Read the model definition and answer for the solid it produces. Units are mm, in the model's axes. Face numbers are marked on the shaded views. A direction names the side the tool comes from. Give positions to 0.01 mm unless a question says otherwise; leave off trailing zeros. Order: outer loops, then holes, each group sorted by start corner. A loop starts at its lowest first (then second) coordinate and runs counter-clockwise, first axis right, second up. Notation, with made-up numbers: (77, 36) - (122, 36) arc R9 cw to (122, 52) - close; hole circle Ø11 at (-28.75, -6.75). An arc over 180 degrees is marked (long way). Use a Markdown table: item, result. Add a question column.
1. A cutting plane is placed at A-A on z = 6.5. Determine the outline of the cut face in (x, y).
2. A cutting plane is placed at B-B on x = -31.5. Determine the outline of the cut face in (y, z), and give its area (3 significant figures).
3. For a pull along X with two mould halves and no side action, classify the marked faces 1, 2 and 3 as released by +X, released by -X, zero draft, split by the parting line, or undercut.
4. A cutting plane is placed at D-D on z = -19.5. Determine the outline of the cut face in (x, y), and give its area (3 significant figures).
5. Consider L1, parallel to X at y = 15, z = 1.5; L2, parallel to Y at x = -53.5, z = -22; L3, parallel to X at y = -77, z = 9.5. Determine where each line is inside the solid, lowest interval first.
6. Flat-ended cylindrical pins translate along their axes: P1, Ø3, axis at y = -39.5, z = 0.5, coming from the -X side; P2, Ø8, axis at x = 3, z = 5, coming from the -Y side; P3, Ø11, axis at y = -70, z = -20.5, coming from the -X side. Find the tip coordinate at first contact, or state that the pin passes through.
7. Which of the six approach directions +Z, -Z, +X, -X, +Y, -Y give full straight-line access (tool end or side, diameter ignored) to the marked faces 4, 5 and 6?
8. A cutting plane is placed at C-C on y = -66.5. Determine the outline of the cut face in (x, z), and give its area (3 significant figures).
```python
from build123d import *

# Parameters (mm, degrees)
F0_W          = 132.9678967595
F0_H          = 40.9901021048
F1_DEPTH      = 35.306
F2_W          = 109.3940883875
F2_H          = 52.1104875952
F3_DEPTH      = 57.15
F4_W          = 66.4839483798
F4_H          = 40.9901021048
F5_DEPTH      = 56.134
F6_W          = 53.8083352149
F6_H          = 26.0552437976
F7_DEPTH      = 59.69
F8_F1_R       = 5.08
F8_F2_R       = 5.08
F9_W          = 99.2340883875
F9_H          = 46.9125229284
F10_DEPTH     = 4.826
F11_W         = 43.6483352149
F11_H         = 56.2114770716
F12_DEPTH     = 4.826
F13_T1_DEPTH  = 56.3324502806
F13_T3_DEPTH  = 0.0774771487
F13_T5_DEPTH  = 68.8181149887
F13_T7_DEPTH  = 55.5857531726
F13_T9_DEPTH  = 115.8081150657
F13_T11_DEPTH = 99.2340883875
F13_T13_DEPTH = 59.5966379941
F13_T19_DEPTH = 68.2698682383
F13_T23_DEPTH = 12.7615922144


# Not quite as in the source:
# - a fillet or chamfer that OpenCascade refuses, or shapes differently, is made with other operations: its cross-section is extruded or revolved along the edge and cut away or added


with BuildPart() as f1:
    # F0 (on Front) → F1 (new body, symmetric)
    with BuildSketch(Plane.XZ):
        with Locations((0.8887089789, -5.8075287379)):
            Rectangle(F0_W, F0_H)
    extrude(amount=F1_DEPTH, both=True)

    # F2 (on face) → F3 (cut)
    with BuildSketch(Plane.XZ.offset(35.306)):
        with Locations((0, 14.6875223145)):
            Rectangle(F2_W, F2_H)
    extrude(amount=-F3_DEPTH, mode=Mode.SUBTRACT)

    # F4 (on face) → F5 (join)
    with BuildSketch(Plane.XZ.offset(35.306)):
        with Locations((34.1306831688, -5.8075287379)):
            Rectangle(F4_W, F4_H)
    extrude(amount=F5_DEPTH)

    # F6 (on face) → F7 (cut)
    with BuildSketch(Plane(origin=(0, -35.306, 0), x_dir=(-1, 0, 0), z_dir=(0, 1, 0))):
        with Locations((-27.7928765863, 1.6599004157)):
            Rectangle(F6_W, F6_H)
    extrude(amount=-F7_DEPTH, mode=Mode.SUBTRACT)

    # F8: fillet of radius 5.08 on 11 edges, made by hand

    # F8_f1
    f8_f1_edges = [f1.edges().sort_by_distance(p)[0] for p in [
        (-54.6970441937, -6.731, -11.3677214831),
        (-54.6970441937, 21.844, 1.6599004157),
        (0, 21.844, -11.3677214831),
        (54.6970441937, -34.798, -11.3677214831),
        (54.6970441937, 21.844, 1.6599004157),
    ]]
    fillet(f8_f1_edges, radius=F8_F1_R)

    # F8_f2
    f8_f2_edges = [f1.edges().sort_by_distance(p)[0] for p in [
        (-54.6970441937, -9.271, 14.6875223145),
        (0, 21.844, 14.6875223145),
        (54.6970441937, -37.338, 14.6875223145),
        (-24.3641676074, -35.306, -11.3677214831),
        (0.8887089789, -63.373, -11.3677214831),
        (25.2528765863, -91.44, -11.3677214831),
        (53.2091466422, -91.44, -9.8798239315),
        (-53.2091466422, -35.306, -9.8798239315),
        (53.2091466422, 20.3561024484, 14.6875223145),
        (-53.2091466422, 20.3561024484, 14.6875223145),
    ]]
    fillet(f8_f2_edges, radius=F8_F2_R)

    # F9 (on face) → F10 (join)
    with BuildSketch(Plane.XY.offset(-11.3677214831)):
        with Locations((0, -6.6922614642)):
            Rectangle(F9_W, F9_H)
    extrude(amount=F10_DEPTH)

    # F11 (on face) → F12 (join)
    with BuildSketch(Plane.XY.offset(-11.3677214831)):
        with Locations((27.7928765863, -58.2542614642)):
            Rectangle(F11_W, F11_H)
    extrude(amount=F12_DEPTH)

    # F13: fillet of radius 5.08 on 6 edges, made by hand

    # F13_s2 → F13_t1 (cut)
    with BuildSketch(Plane.YZ.offset(-6.7154060868)):
        with BuildLine():
            ThreePointArc((-81.2863539737, -6.5417214831), (-84.7875023567, -7.9409117896), (-86.36, -11.3677214831))
            Line((-86.36, -11.3677214831), (-86.36, -6.5417214831))
            Line((-86.36, -6.5417214831), (-81.2863539737, -6.5417214831))
        make_face()
    extrude(amount=F13_T1_DEPTH, mode=Mode.SUBTRACT)

    # F13_s4 → F13_t3 (cut)
    with BuildSketch(Plane.XZ.offset(30.1485229284)):
        with BuildLine():
            ThreePointArc((11.0423550052, -6.5417214831), (7.5412066221, -7.9409117896), (5.9687089789, -11.3677214831))
            Line((5.9687089789, -11.3677214831), (5.9687089789, -6.5417214831))
            Line((5.9687089789, -6.5417214831), (11.0423550052, -6.5417214831))
        make_face()
    extrude(amount=F13_T3_DEPTH, mode=Mode.SUBTRACT)

    # F13_s6 → F13_t5 (cut)
    with BuildSketch(Plane.XZ.offset(30.226000077)):
        with BuildLine():
            ThreePointArc((11.0423550052, -6.5417214831), (7.5412066221, -7.9409117896), (5.9687089789, -11.3677214831))
            Line((5.9687089789, -11.3677214831), (5.9687089789, -6.5417214831))
            Line((5.9687089789, -6.5417214831), (11.0423550052, -6.5417214831))
        make_face()
    extrude(amount=F13_T5_DEPTH, mode=Mode.SUBTRACT)

    # F13_s8 → F13_t7 (cut)
    with BuildSketch(Plane.YZ.offset(-49.6170441937)):
        with BuildLine():
            ThreePointArc((-25.0748769021, -6.5417214831), (-28.5760252851, -7.9409117896), (-30.1485229284, -11.3677214831))
            Line((-30.1485229284, -11.3677214831), (-30.1485229284, -6.5417214831))
            Line((-30.1485229284, -6.5417214831), (-25.0748769021, -6.5417214831))
        make_face()
    extrude(amount=F13_T7_DEPTH, mode=Mode.SUBTRACT)

    # F13_s10 → F13_t9 (cut)
    with BuildSketch(Plane.XZ.offset(-16.764)):
        with BuildLine():
            ThreePointArc((44.5433981675, -6.5417214831), (48.0445465505, -7.9409117896), (49.6170441937, -11.3677214831))
            Line((49.6170441937, -11.3677214831), (49.6170441937, -6.5417214831))
            Line((49.6170441937, -6.5417214831), (44.5433981675, -6.5417214831))
        make_face()
    extrude(amount=F13_T9_DEPTH, mode=Mode.SUBTRACT)

    # F13_s12 → F13_t11 (cut)
    with BuildSketch(Plane.YZ.offset(-49.6170441937)):
        with BuildLine():
            ThreePointArc((16.764, -11.3677214831), (15.1915023567, -7.9409117896), (11.6903539737, -6.5417214831))
            Line((11.6903539737, -6.5417214831), (16.764, -6.5417214831))
            Line((16.764, -6.5417214831), (16.764, -11.3677214831))
        make_face()
    extrude(amount=F13_T11_DEPTH, mode=Mode.SUBTRACT)

    # F13_s14 → F13_t13 (cut)
    with BuildSketch(Plane.XZ.offset(-16.764)):
        with BuildLine():
            ThreePointArc((-44.5433981675, -6.5417214831), (-48.0445465505, -7.9409117896), (-49.6170441937, -11.3677214831))
            Line((-49.6170441937, -11.3677214831), (-49.6170441937, -6.5417214831))
            Line((-49.6170441937, -6.5417214831), (-44.5433981675, -6.5417214831))
        make_face()
    extrude(amount=F13_T13_DEPTH, mode=Mode.SUBTRACT)


with BuildPart() as f13_tool17:
    # F13_s18 → F13_t19 (new body)
    with BuildSketch(Plane.YZ.offset(-49.6170441937)):
        with BuildLine():
            ThreePointArc((-25.0748769021, -6.5417214831), (-28.5760252851, -7.9409117896), (-30.1485229284, -11.3677214831))
            Line((-30.1485229284, -11.3677214831), (-30.1485229284, -6.5417214831))
            Line((-30.1485229284, -6.5417214831), (-25.0748769021, -6.5417214831))
        make_face()
    extrude(amount=F13_T19_DEPTH)

    split(bisect_by=Plane.YZ.offset(5.9687089789), keep=Keep.TOP)


with BuildPart() as f13_tool21:
    # F13_s22 → F13_t23 (new body)
    with BuildSketch(Plane.XZ.offset(17.4644078627)):
        with BuildLine():
            ThreePointArc((11.0423550052, -6.5417214831), (7.5412066221, -7.9409117896), (5.9687089789, -11.3677214831))
            Line((5.9687089789, -11.3677214831), (5.9687089789, -6.5417214831))
            Line((5.9687089789, -6.5417214831), (11.0423550052, -6.5417214831))
        make_face()
    extrude(amount=F13_T23_DEPTH)

    split(bisect_by=Plane.XZ.offset(30.1485229284), keep=Keep.BOTTOM)


with BuildPart() as f13_tool17_1:
    add(f13_tool17.part)

    # F13_t25: intersect F13_tool21
    add(f13_tool21.part, mode=Mode.INTERSECT)


with BuildPart() as f1_1:
    add(f1.part)

    # F13_t15: cut F13_tool17
    add(f13_tool17_1.part, mode=Mode.SUBTRACT)


solid = f1_1.part
```
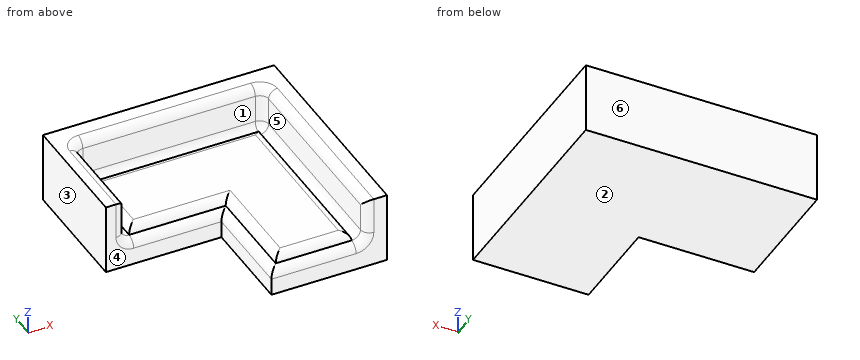
Output values:
| question | item | result |
|---|---|---|
| 1 | outline | (-65.6, -35.31) - (-59.78, -35.31) arc R5.08 ccw to (-54.7, -30.23) - (-54.7, 16.76) arc R5.08 cw to (-49.62, 21.84) - (49.62, 21.84) arc R5.08 cw to (54.7, 16.76) - (54.7, -86.36) arc R5.08 ccw to (59.78, -91.44) - (67.37, -91.44) - (67.37, 35.31) - (-65.6, 35.31) - close |
| 2 | outline | (-35.31, -26.3) - (35.31, -26.3) - (35.31, 14.69) - (26.92, 14.69) arc R5.08 ccw to (21.84, 9.61) - (21.84, -6.29) arc R5.08 cw to (16.76, -11.37) arc R5.08 ccw to (11.69, -6.54) - (-25.07, -6.54) arc R5.08 ccw to (-30.15, -11.37) - (-30.23, -11.37) arc R5.08 ccw to (-35.31, -16.45) - close |
| 2 | area | 1,620 mm² |
| 3 | face 1 | undercut |
| 3 | face 2 | zero draft |
| 3 | face 3 | released by -X |
| 4 | outline | (-65.6, -35.31) - (0.89, -35.31) - (0.89, -91.44) - (67.37, -91.44) - (67.37, 35.31) - (-65.6, 35.31) - close |
| 4 | area | 13,100 mm² |
| 5 | L1 | -65.6 to -54.7, 54.7 to 67.37 |
| 5 | L2 | -35.31 to 35.31 |
| 5 | L3 | 54.7 to 67.37 |
| 6 | P1 | x = 54.7 |
| 6 | P2 | y = 21.84 |
| 6 | P3 | x = 0.89 |
| 7 | face 4 | +Z, -Z, -X, -Y |
| 7 | face 5 | +Z, -Y |
| 7 | face 6 | +Z, -Z, +X, -X, +Y |
| 8 | outline | (0.89, -26.3) - (67.37, -26.3) - (67.37, 14.69) - (59.78, 14.69) arc R5.08 ccw to (54.7, 9.61) - (54.7, -6.29) arc R5.08 cw to (49.62, -11.37) arc R5.08 ccw to (44.54, -6.54) - (11.04, -6.54) arc R5.08 ccw to (5.97, -11.37) arc R5.08 ccw to (0.89, -16.45) - close |
| 8 | area | 1,520 mm² |
